Verification items for the finished model (mm, model axes). A direction names the side the tool comes from. Give positions to 0.01 mm unless a question says otherwise; leave off trailing zeros. Write each loop counter-clockwise with the first axis right and the second up, starting at its lowest first coordinate (ties: lowest second). Pieces come first, ordered by that corner, then holes.
from build123d import *

# Parameters (mm, degrees)
SKETCH1_R           = 5
BOSS_EXTRUDE1_DEPTH = 30
SKETCH4_R           = 7.5
BOSS_EXTRUDE3_DEPTH = 3
SKETCH5_W           = 3
SKETCH5_H           = 10
BOSS_EXTRUDE4_DEPTH = 7
SKETCH6_R           = 2
CUT_EXTRUDE2_DEPTH  = 7
FILLET1_R           = 1
FILLET2_R           = 5


with BuildPart() as part:
    # Sketch1 → Boss-Extrude1 (new body)
    with BuildSketch(Plane(origin=(0, 0, 0), x_dir=(1, 0, 0), z_dir=(0, 1, 0))):
        with Locations(Location((0, 0, 0), (0, 0, 270))):
            Circle(SKETCH1_R)
    extrude(amount=BOSS_EXTRUDE1_DEPTH)

    # Sketch4 → Boss-Extrude3 (add)
    with BuildSketch(Plane(origin=(0, 30, 0), x_dir=(1, 0, 0), z_dir=(0, 1, 0))):
        with Locations(Location((0, 0, 0), (0, 0, 270))):
            Circle(SKETCH4_R)
    extrude(amount=BOSS_EXTRUDE3_DEPTH)

    # Sketch5 → Boss-Extrude4 (add)
    with BuildSketch(Plane(origin=(0, 33, 0), x_dir=(1, 0, 0), z_dir=(0, 1, 0))):
        Rectangle(SKETCH5_W, SKETCH5_H)
    extrude(amount=BOSS_EXTRUDE4_DEPTH)

    # Sketch6 → Cut-Extrude2 (cut)
    with BuildSketch(Plane(origin=(1.5, 0, 0), x_dir=(0, 0, -1), z_dir=(1, 0, 0))):
        with Locations((0, 37)):
            Circle(SKETCH6_R)
    extrude(amount=-CUT_EXTRUDE2_DEPTH, mode=Mode.SUBTRACT)

    # Fillet1
    fillet1_edges = [part.edges().sort_by_distance(p)[0] for p in [
        (1.5, 33, 0),
        (0, 33, -5),
        (-1.5, 33, 0),
        (0, 33, 5),
        (0, 30, -5),
        (0, 30, -7.5),
        (0, 33, -7.5),
    ]]
    fillet(fillet1_edges, radius=FILLET1_R - 0.0001)  # a hair under: the kernel refuses the full size

    # Fillet2
    fillet2_edges = [part.edges().sort_by_distance(p)[0] for p in [
        (0, 40, -5),
        (0, 40, 5),
    ]]
    fillet(fillet2_edges, radius=FILLET2_R - 0.0001)  # a hair under: the kernel refuses the full size


solid = part.part
Item 1: Sectioned sample at C-C on y = 4.5. Record the cut outline in (x, z).
Answer key:
outline: circle Ø10 at (0, 0)
Item 2: Depth check by flat-ended pin: pin 1 (8 mm diameter, centred on y = 21.5, z = 4.5, fed in from -X); pin 2 (5 mm diameter, centred on y = 37, z = 0.5, fed in from +X); pin 3 (3 mm diameter, centred on x = -4, z = 2, fed in from +Y). Enter the tip coordinate at first touch or a pass-through.
Answer key:
pin 1: stops at x = -4.97
pin 2: stops at x = 1.5
pin 3: stops at y = 33
Item 3: Scan lines: line 1 along Y through (x, z) = (-0.25, 0); line 2 along Y through (x, z) = (-0.5, 1.5); line 3 along X through (y, z) = (19.5, -3.5). Record each from-to range of solid material in increasing order.
Answer key:
line 1: y = 0 to 35, 39 to 40
line 2: y = 0 to 35.68, 38.32 to 39.77
line 3: x = -3.57 to 3.57
Item 4: Release check for a two-part mould opening along Z. For faces 4 (the face through (-3, 33, 0)), 5 (the face through (0, 34.5, 5)), 6 (the face through (0, 33.2, -5.4)), 7 (the face through (0, 35, 0)) record: released by +Z, released by -Z, zero draft, split by the parting line, or undercut.
Answer key:
face 4: zero draft
face 5: released by +Z
face 6: released by -Z
face 7: undercut
Item 5: Set-up check for faces 1 (the face through (1.5, 35, -1)), 2 (the face through (-4.88, 14.3, -1.08)), 3 (the face through (0, 34.5, -5)): record each of +Z, -Z, +X, -X, +Y, -Y from which the full face is reachable in a straight line by a thin tool's end or side.
Answer key:
face 1: +Z, -Z, +X, +Y
face 2: -Y
face 3: -Z, +X, -X, +Y
Item 6: Sectioned sample at B-B on y = 36.5. Record the cut outline in (x, z), then the cut area to 3 significant figures.
Answer key:
outline: (-1.5, -4.77) - (1.5, -4.77) - (1.5, -1.94) - (-1.5, -1.94) - close; (-1.5, 1.94) - (1.5, 1.94) - (1.5, 4.77) - (-1.5, 4.77) - close
area: 17.0 mm2
